Drawing for the job (mm, zero at the part's lowest x, y, z). A direction names the side the tool comes from. Coordinates: 2 decimals unless noted, no trailing zeros. Write each loop counter-clockwise with the first axis right and the second up, starting at its lowest first coordinate (ties: lowest second). Pieces come first, ordered by that corner, then holes. Notation, with made-up numbers: (45, 51.25) -> (75, 51.25) arc R4 cw to (75, 58.25) -> close; hole circle Ø4 at (88, 74). An arc over 180 degrees is marked (long way). Write item = value, one per line. Start each with the question number.
Q1. Pull direction Z, two halves, no side cores. Call the marked faces 3, 4, 5 and 6: released by +Z, released by -Z, zero draft, split by the parting line, or undercut.
Q2. Pin check, flat tips, straight feed: P1, Ø5, axis at x = 42.5, y = 6.5, coming from the +Z side (1 decimal); P2, Ø5, axis at x = 35, y = 3, coming from the -Z side; P3, Ø5, axis at y = 8, z = 82, coming from the -X side; P4, Ø5, axis at x = 60, z = 49.5, coming from the +Y side. Stop position of each tip, or through.
Q3. Probe line 1 (X direction, y = 3.75, z = 60); line 2 (Z direction, x = 41, y = 8.5); line 3 (X direction, y = 4, z = 82.5). List the from-to ranges inside material, lowest first.
Q4. Band-saw the part on A-A, the plane z = 60. List the corners of the cut face in (x, y), plus the area to 3 significant figures.
Q5. Band-saw the part on B-B, the plane x = 60. List the corners of the cut face in (y, z).
Q6. Band-saw the part on C-C, the plane y = 4.5. Give the number of separate pieces and of enclosed holes in the cut face, plus the area to 3 significant figures.
Q7. Band-saw the part on D-D, the plane z = 10. List the corners of the cut face in (x, y).
Q8. Tool access for the marked faces 1 and 2: list every direction of +Z, -Z, +X, -X, +Y, -Y with a clear straight run to the whole face (end or side of a thin tool).
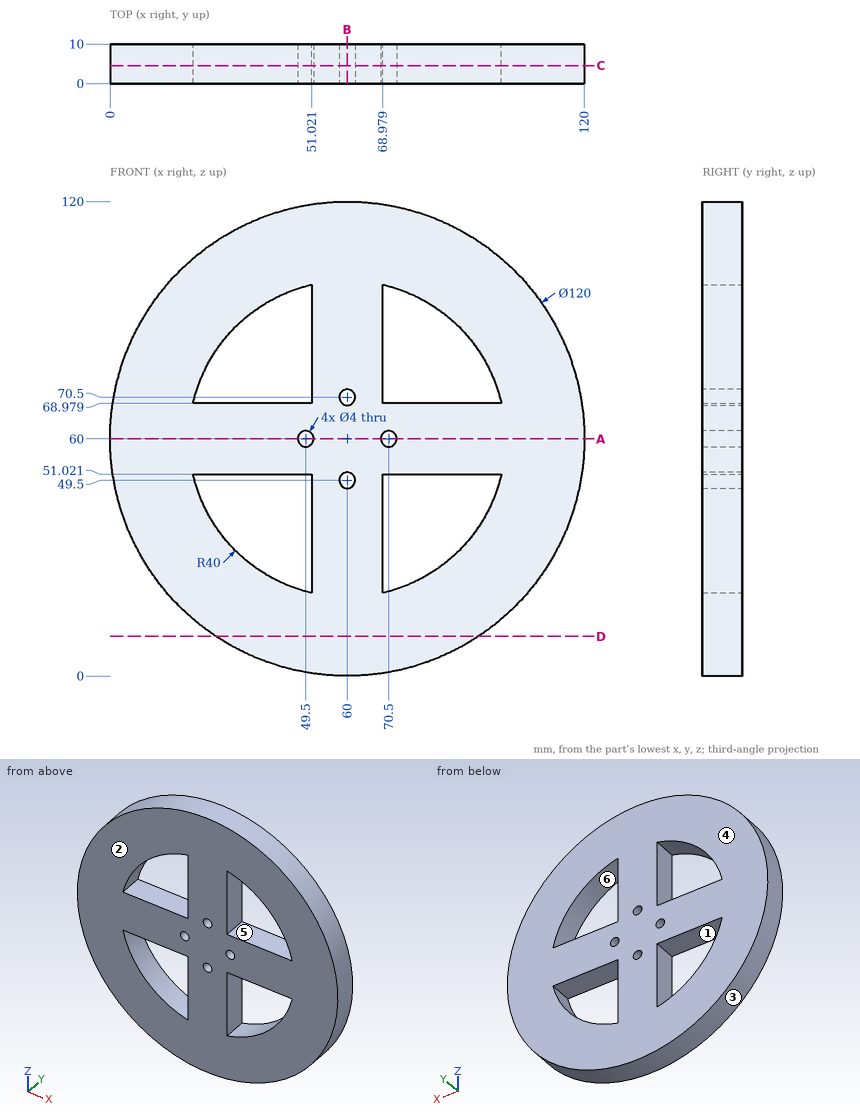
Ans:
q1.face_3 = split by the parting line
q1.face_4 = zero draft
q1.face_5 = undercut
q1.face_6 = undercut
q2.P1 = 118.1
q2.P2 = 4.38
q2.P3 = 3.26
q2.P4 = 10
q3.line_1 = 0 to 47.5, 51.5 to 68.5, 72.5 to 120
q3.line_2 = 3.09 to 24.8, 51.02 to 68.98, 95.2 to 116.91
q3.line_3 = 4.38 to 26.93, 51.02 to 68.98, 93.07 to 115.62
q4.outline = (0, 0) -> (47.5, 0) -> (47.5, 10) -> (0, 10) -> close; (51.5, 0) -> (68.5, 0) -> (68.5, 10) -> (51.5, 10) -> close; (72.5, 0) -> (120, 0) -> (120, 10) -> (72.5, 10) -> close
q4.area = 1,120 mm2
q5.outline = (0, 0) -> (10, 0) -> (10, 47.5) -> (0, 47.5) -> close; (0, 51.5) -> (10, 51.5) -> (10, 68.5) -> (0, 68.5) -> close; (0, 72.5) -> (10, 72.5) -> (10, 120) -> (0, 120) -> close
q6.separate_pieces = 1
q6.enclosed_holes = 8
q6.area = 8,760 mm2
q7.outline = (26.83, 0) -> (93.17, 0) -> (93.17, 10) -> (26.83, 10) -> close
q8.face_1 = +Y, -Y
q8.face_2 = +Z, -Z, +X, -X, -Y
